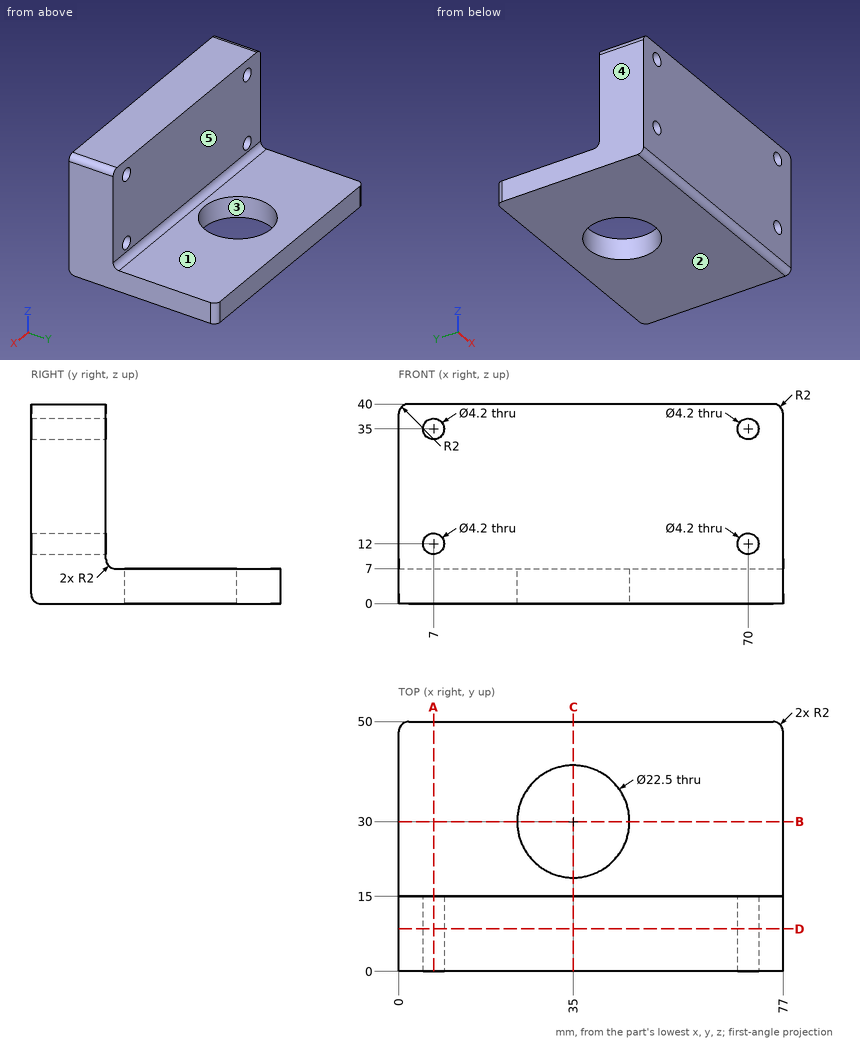
The figure shows three views and two pictorial views of one solid part (mm, origin at its lowest corner). Answer the questions. A direction names the side the tool comes from. Coordinates: 2 decimals unless noted, no trailing zeros. Loops run counter-clockwise (first coordinate to the right, second up) from the corner with the lowest first, then second, coordinate; pieces in that order, holes last.
1) Find section C-C on x = 35. Write down the section's boundary in (y, z).
2) Find section D-D on y = 8.5. Write down the section's boundary in (x, z), then the cut area to 3 significant figures.
3) Find the intervals of material crossed by L1, parallel to Z at x = 7, y = 11.75; L2, parallel to X at y = 6, z = 12; L3, parallel to X at y = 11, z = 10.5, in increasing order.
4) Find section A-A on x = 7. Write down the section's boundary in (y, z).
5) Determine the mould class of the marked faces 3, 4 and 5 for opening direction Y: pulls with the +Y half, pulls with the -Y half, needs draft (parallel to the pull), parting line crosses it, or undercut.
6) A tool of negligible diameter and unlimited length cuts with its end or side. For the marked faces 1 and 2, from which of +Z, -Z, +X, -X, +Y, -Y can it reach the whole face along a straight path? Write none if from no direction.
7) Flat-ended cylindrical pins translate along their axes: pin 1 Ø4 at (x, z) = (7, 12) entering from +Y; pin 2 Ø1 at (x, z) = (64, 35.5) entering from +Y. Find the tip coordinate at first contact, or state that the pin passes through.
8) Find section B-B on y = 30. Write down the section's boundary in (x, z).
Values:
1. outline: (0, 2) arc R2 ccw to (2, 0) - (18.75, 0) - (18.75, 7) - (17, 7) arc R2 cw to (15, 9) - (15, 40) - (0, 40) - close; (41.25, 0) - (50, 0) - (50, 7) - (41.25, 7) - close
2. outline: (0, 0) - (77, 0) - (77, 38) arc R2 ccw to (75, 40) - (2, 40) arc R2 ccw to (0, 38) - close; hole circle Ø4.2 at (7, 12); hole circle Ø4.2 at (7, 35); hole circle Ø4.2 at (70, 12); hole circle Ø4.2 at (70, 35)
2. area: 3,020 mm2
3. L1: z = 0 to 9.9, 14.1 to 32.9, 37.1 to 40
3. L2: x = 0 to 4.9, 9.1 to 67.9, 72.1 to 77
3. L3: x = 0 to 5.53, 8.47 to 68.53, 71.47 to 77
4. outline: (0, 2) arc R2 ccw to (2, 0) - (50, 0) - (50, 7) - (17, 7) arc R2 cw to (15, 9) - (15, 9.9) - (0, 9.9) - close; (0, 14.1) - (15, 14.1) - (15, 32.9) - (0, 32.9) - close; (0, 37.1) - (15, 37.1) - (15, 40) - (0, 40) - close
5. face 3: undercut
5. face 4: needs draft
5. face 5: pulls with the +Y half
6. face 1: +Z, +X, -X, +Y
6. face 2: -Z, +X, -X, +Y, -Y
7. pin 1: passes through
7. pin 2: stops at y = 15
8. outline: (0, 0) - (23.75, 0) - (23.75, 7) - (0, 7) - close; (46.25, 0) - (77, 0) - (77, 7) - (46.25, 7) - close
